Here's how the part is built. I have some questions about the finished solid (model axes, mm). Face numbers are marked on the shaded views. A direction names the side the tool comes from. Round coordinates to 2 decimals unless told otherwise and drop trailing zeros. Write each loop counter-clockwise with the first axis right and the second up, starting at its lowest first coordinate (ties: lowest second). Pieces come first, ordered by that corner, then holes. Notation, with made-up numbers: (-39, -34) -> (-21, -34) arc R15 ccw to (-21, -22) -> close; hole circle Ø3 at (44.25, 23). An arc over 180 degrees is marked (long way). Put each result on its own line as item: value. Start each with the question number.
1. Suppose I cut it at D-D (x = 0.5). Please give me the cut outline in (y, z).
2. I need wall thicknesses on probe 1 along Z at (x, y) = (11, 6.25); probe 2 along Z at (x, y) = (0, 8.5); probe 3 along Z at (x, y) = (8.5, 5.75). Which ranges of each line are inside material? Lowest first, please. Write a range as from..to.
3. For pin 1 (7 mm diameter, centred on x = -5.5, z = 5, fed in from -Y); pin 2 (6.5 mm diameter, centred on y = 3, z = 8.5, fed in from +X); pin 3 (2.5 mm diameter, centred on y = 10, z = 0, fed in from +X), each with a flat end and sliding along its axis, tell me the tip position at first contact or that it passes through.
4. Suppose I cut it at A-A (z = 0). Please give me the cut outline in (x, y).
5. Which directions (+Z, -Z, +X, -X, +Y, -Y) give clear straight access to the entire face, cutting with the end or side of a thin tool? Please do the marked faces 1, 2 and 3.
6. We'd pull the mould along Y, two halves only. Please class the marked faces 4, 5 and 6: +Y half, -Y half, draft (parallel to the pull), parting line (faces both ways), or undercut.
7. Suppose I cut it at C-C (z = 6). Please give me the cut outline in (x, y).
8. Suppose I cut it at B-B (y = 2). Please give me the cut outline in (x, z), then the cut area to 3 significant figures.
```python
from build123d import *

# Parameters (mm, degrees)
SKETCH1_W           = 28.6
SKETCH1_H           = 5
BOSS_EXTRUDE1_DEPTH = 14
CUT_EXTRUDE1_DEPTH  = 4
SKETCH5_R           = 2.5
BOSS_EXTRUDE4_DEPTH = 4
BOSS_EXTRUDE5_DEPTH = 28.6
SKETCH7_W           = 20
SKETCH7_H           = 3
BOSS_EXTRUDE6_DEPTH = 10
FILLET1_R           = 10


with BuildPart() as part:
    # Sketch1 → Boss-Extrude1 (new body)
    with BuildSketch(Plane(origin=(0, 0, 0), x_dir=(1, 0, 0), z_dir=(0, 1, 0))):
        Rectangle(SKETCH1_W, SKETCH1_H)
    extrude(amount=BOSS_EXTRUDE1_DEPTH)

    # Sketch2 → Cut-Extrude1 (cut)
    with BuildSketch(Plane(origin=(14.3, 0, 0), x_dir=(0, 0, -1), z_dir=(1, 0, 0))):
        with BuildLine():
            Line((-1.5875, 5.25), (-1.5875, 11.4))
            ThreePointArc((-1.5875, 11.4), (0, 12.9875), (1.5875, 11.4))
            Line((1.5875, 11.4), (1.5875, 5.25))
            ThreePointArc((1.5875, 5.25), (0, 3.6625), (-1.5875, 5.25))
        make_face()
    cut_extrude1 = extrude(amount=-CUT_EXTRUDE1_DEPTH, mode=Mode.SUBTRACT)

    # Sketch5 → Boss-Extrude4 (add)
    with BuildSketch(Plane.XZ):
        with Locations(Location((0, 0, 0), (0, 0, 270))):
            Circle(SKETCH5_R)
    extrude(amount=BOSS_EXTRUDE4_DEPTH)

    # Sketch6 → Boss-Extrude5 (add)
    with BuildSketch(Plane(origin=(14.3, 0, 0), x_dir=(0, 0, -1), z_dir=(1, 0, 0))):
        Polygon((-2.5, 14), (-6.5, 14), (-6.5, 12), (-2.5, 8), align=None)
    extrude(amount=-BOSS_EXTRUDE5_DEPTH)

    # Mirror1: Cut-Extrude1 across plane
    add(cut_extrude1.mirror(Plane(origin=(0, 0, 0), x_dir=(0, 0, 1), z_dir=(1, 0, 0))), mode=Mode.SUBTRACT)

    # Sketch7 → Boss-Extrude6 (add)
    with BuildSketch(Plane.ZY.offset(14.3)):
        with Locations((12.5, 1.5)):
            Rectangle(SKETCH7_W, SKETCH7_H)
    extrude(amount=-BOSS_EXTRUDE6_DEPTH)

    # Fillet1
    # the kernel refuses this fillet: 10 mm, written as the material it adds along each edge
    with BuildSketch(Plane(origin=(-14.3, 3, 2.5), x_dir=(0, 1, 0), z_dir=(1, 0, 0))) as fillet1_piece_1:
        with BuildLine():
            CenterArc((10, 8.660254038), FILLET1_R, 180, 60)
            Line((0, 8.660254038), (-0.2, 8.660254038))
            Line((-0.2, 8.660254038), (-0.2, 0))
            Line((-0.2, 0), (0, -0.2))
            ThreePointArc((0, -0.2), (2.5, -0.2), (4.9, -0.173205081))
            Line((4.9, -0.173205081), (5, 0))
        make_face()
    extrude(amount=10)


solid = part.part
```
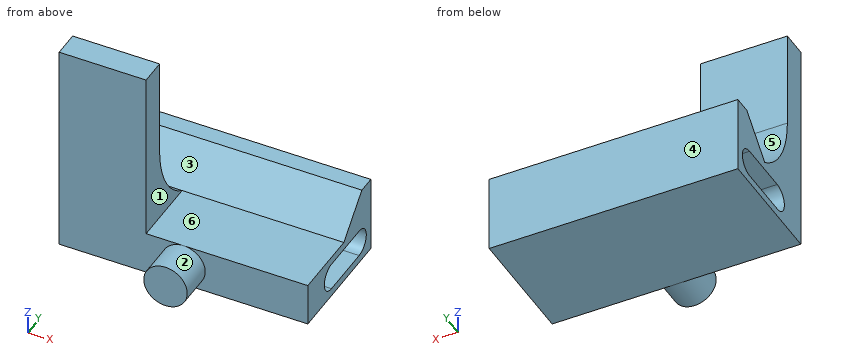
Verdict:
1. outline: (-4, -2.45) -> (0, -2.45) -> (0, -2.5) -> (14, -2.5) -> (14, 6.5) -> (12, 6.5) -> (8, 2.5) -> (0, 2.5) -> (0, 2.45) -> (-4, 2.45) -> close
2. probe 1: z = -2.5..-1.59, 1.59..2.5
2. probe 2: z = -2.5..3
2. probe 3: z = -2.5..2.5
3. pin 1: stops at y = 0
3. pin 2: stops at x = -4.3
3. pin 3: stops at x = 10.3
4. outline: (-14.3, 0) -> (-2.5, 0) -> (-2.5, -4) -> (2.5, -4) -> (2.5, 0) -> (14.3, 0) -> (14.3, 3.66) -> (10.3, 3.66) -> (10.3, 12.99) -> (14.3, 12.99) -> (14.3, 14) -> (-14.3, 14) -> (-14.3, 12.99) -> (-10.3, 12.99) -> (-10.3, 3.66) -> (-14.3, 3.66) -> close
5. face 1: +Z, +X, -Y
5. face 2: -Y
5. face 3: +Z, +X, -X
6. face 4: +Y half
6. face 5: undercut
6. face 6: draft
7. outline: (-14.3, 0) -> (-4.3, 0) -> (-4.3, 4.43) -> (-14.3, 4.43) -> close; (-14.3, 11.5) -> (14.3, 11.5) -> (14.3, 14) -> (-14.3, 14) -> close
8. outline: (-14.3, -2.5) -> (14.3, -2.5) -> (14.3, 2.5) -> (-4.3, 2.5) -> (-4.3, 22.5) -> (-14.3, 22.5) -> close
8. area: 343 mm^2
